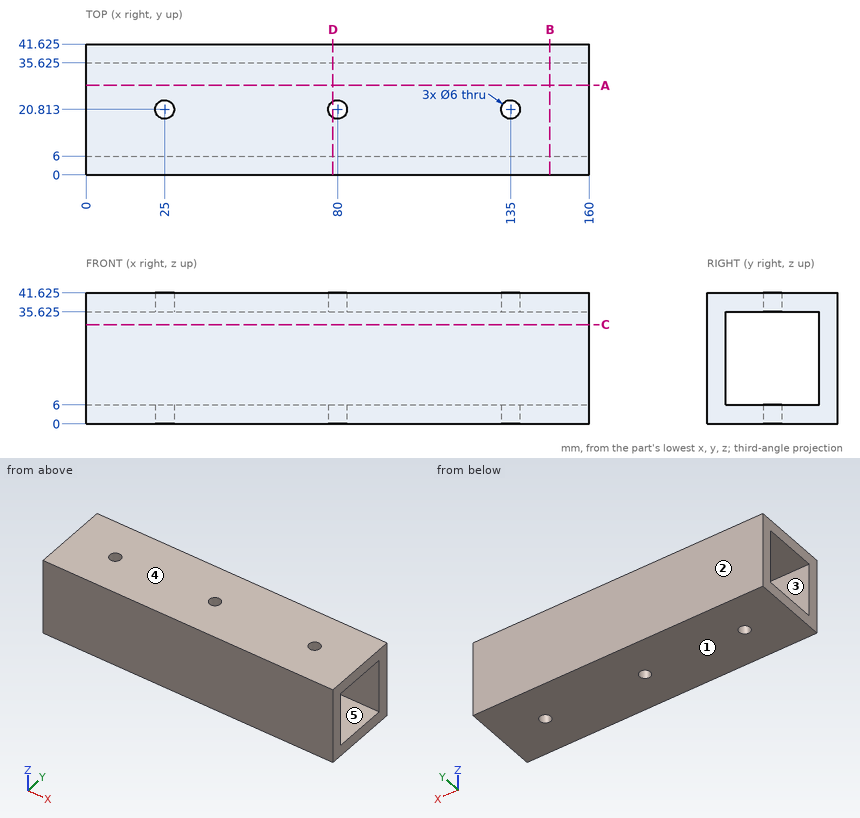
Part print with two shaded views. Sizes in mm from the minimum x, y, z corner. A direction names the side the tool comes from. Coordinates: 2 decimals unless noted, no trailing zeros. Write each loop counter-clockwise with the first axis right and the second up, starting at its lowest first coordinate (ties: lowest second). Pieces come first, ordered by that corner, then holes.
(1) 3-axis set-ups, long thin cutter, end or side, ignore diameter. For the marked faces 4 and 5: which of +Z, -Z, +X, -X, +Y, -Y reach the whole face in a straight line?
(2) Cut at A-A on y = 28.5. List the corners of the cut face in (x, z) (1 decimal).
(3) Cut at D-D on x = 78.5. List the corners of the cut face in (y, z) (1 decimal).
(4) Cut at B-B on x = 147.5. List the corners of the cut face in (y, z) (1 decimal), and give its area (3 significant figures).
(5) Drill centre lines: line 1 (Y direction, x = 19, z = 22) (1 decimal); line 2 (Y direction, x = 135, z = 39.1) (1 decimal). Where is each one in solid material? Low to high.
(6) Mould opens along Z. For the marked faces 1, 2 and 3 say: pulls with the +Z half, pulls with the -Z half, needs draft (parallel to the pull), parting line crosses it, or undercut.
Working result:
1. face 4: +Z, +X, -X, +Y, -Y
1. face 5: +X, -X
2. outline: (0, 0) - (160, 0) - (160, 6) - (0, 6) - close; (0, 35.6) - (160, 35.6) - (160, 41.6) - (0, 41.6) - close
3. outline: (0, 0) - (18.2, 0) - (18.2, 6) - (6, 6) - (6, 35.6) - (18.2, 35.6) - (18.2, 41.6) - (0, 41.6) - close; (23.4, 0) - (41.6, 0) - (41.6, 41.6) - (23.4, 41.6) - (23.4, 35.6) - (35.6, 35.6) - (35.6, 6) - (23.4, 6) - close
4. outline: (0, 0) - (41.6, 0) - (41.6, 41.6) - (0, 41.6) - close; hole (6, 6) - (35.6, 6) - (35.6, 35.6) - (6, 35.6) - close
4. area: 855 mm2
5. line 1: y = 0 to 6, 35.6 to 41.6
5. line 2: y = 0 to 17.8, 23.8 to 41.6
6. face 1: pulls with the -Z half
6. face 2: needs draft
6. face 3: undercut
